from build123d import *

# Parameters (mm, degrees)
EXTRUDE_1_DEPTH     = 20
SKETCH_3_R          = 14
CUT_EXTRUDE_1_DEPTH = 20
SKETCH_4_R          = 3
CUT_EXTRUDE_2_DEPTH = 22.516585743
EXTRUDE_2_DEPTH     = 20
SKETCH_7_R          = 13.5
CUT_EXTRUDE_3_DEPTH = 28
SKETCH_8_R          = 3
CUT_EXTRUDE_4_DEPTH = 20
SKETCH_9_R          = 7.5
SKETCH_9_R_2        = 3
CUT_EXTRUDE_5_DEPTH = 20


# Read off the part's stored shape, not the designer's step: 填料-伸長1
with BuildPart() as part:
    # 填料-伸長1 outline → 填料-伸長1 (new body)
    with BuildSketch(Plane(origin=(0, 0, 0), x_dir=(0, 0, -1), z_dir=(1, 0, 0))):
        Polygon((-4019.675958787, 200.25160655), (-4018.512862627, 177.765080788), (-3958.59296353, 180.864385914), (-3959.75605969, 203.350911676), align=None)
    extrude(amount=EXTRUDE_1_DEPTH)

    # 草圖3 → 除料-伸長1 (cut)
    with BuildSketch(Plane.ZY):
        with Locations((3988.552913079, 179.314733351)):
            Circle(SKETCH_3_R)
    extrude(amount=-CUT_EXTRUDE_1_DEPTH, mode=Mode.SUBTRACT)

    # 草圖4 → 除料-伸長2 (cut)
    with BuildSketch(Plane(origin=(0, 407.076792548, 21.055696166), x_dir=(1, 0, 0), z_dir=(0, 0.9986649849421085, 0.051655085428040495))):
        with Locations(Location((10, -3950.965617011, 0), (0, 0, 270))):
            Circle(SKETCH_4_R)
    cut_extrude_2 = extrude(amount=-CUT_EXTRUDE_2_DEPTH, mode=Mode.SUBTRACT)

    # 鏡射1: 除料-伸長2 across plane
    add(cut_extrude_2.mirror(Plane(origin=(0, -205.275533435, 3968.660313072), x_dir=(1, 0, 0), z_dir=(0, 0.05165508542804326, -0.9986649849421085))), mode=Mode.SUBTRACT)


with BuildPart() as body_2:
    # 草圖6 → 填料-伸長2 (new body)
    with BuildSketch(Plane(origin=(0, 0, 0), x_dir=(0, 0, -1), z_dir=(1, 0, 0))):
        with BuildLine():
            Line((-4017.894989071, 165.819525376), (-4018.512862627, 177.765080788))
            Line((-4018.512862627, 177.765080788), (-3958.59296353, 180.864385914))
            Line((-3958.59296353, 180.864385914), (-3957.975089975, 168.918830502))
            ThreePointArc((-3957.975089975, 168.918830502), (-3987.51981137, 159.341433652), (-4017.894989071, 165.819525376))
        make_face()
    extrude(amount=EXTRUDE_2_DEPTH)

    # 草圖7 → 除料-伸長3 (cut)
    with BuildSketch(Plane.ZY):
        with Locations((3988.552913079, 179.314733351)):
            Circle(SKETCH_7_R)
    extrude(amount=-CUT_EXTRUDE_3_DEPTH, mode=Mode.SUBTRACT)

    # 草圖8 → 除料-伸長4 (cut)
    with BuildSketch(Plane(origin=(0, 384.590266786, 19.892600006), x_dir=(1, 0, 0), z_dir=(0, 0.9986649849421085, 0.05165508542804074))):
        with Locations(Location((10, -3996.965617011, 0), (0, 0, 270))):
            Circle(SKETCH_8_R)
    cut_extrude_4 = extrude(amount=-CUT_EXTRUDE_4_DEPTH, mode=Mode.SUBTRACT)

    # 草圖9 → 除料-伸長5 (cut)
    with BuildSketch(Plane(origin=(0, 372.644711374, 19.27472645), x_dir=(1, 0, 0), z_dir=(0, 0.9986649849421085, 0.05165508542804074))):
        with Locations((10, -3996.965617011)):
            Circle(SKETCH_9_R)
        with Locations(Location((10, -3996.965617011, 0), (0, 0, 270))):
            Circle(SKETCH_9_R_2, mode=Mode.SUBTRACT)
    cut_extrude_5 = extrude(amount=-CUT_EXTRUDE_5_DEPTH, mode=Mode.SUBTRACT)

    # 鏡射4: 除料-伸長4, 除料-伸長5 across plane
    add(cut_extrude_4.mirror(Plane(origin=(0, -205.275533435, 3968.660313072), x_dir=(1, 0, 0), z_dir=(0, 0.05165508542804326, -0.9986649849421085))), mode=Mode.SUBTRACT)
    add(cut_extrude_5.mirror(Plane(origin=(0, -205.275533435, 3968.660313072), x_dir=(1, 0, 0), z_dir=(0, 0.05165508542804326, -0.9986649849421085))), mode=Mode.SUBTRACT)


solid = body_2.part
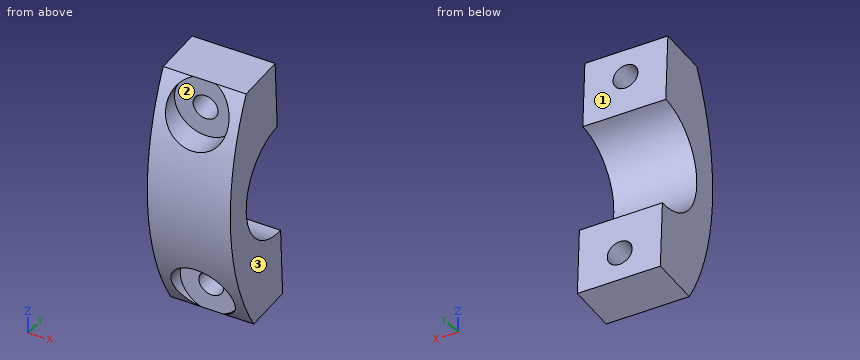
Could you check a few things on this model? Use its own coordinates, in mm. Face numbers are marked on the shaded views. Give positions to 0.01 mm unless a question says otherwise; leave off trailing zeros. Order: outer loops, then holes, each group sorted by start corner. A loop starts at its lowest first (then second) coordinate and runs counter-clockwise, first axis right, second up. Notation, with made-up numbers: (22.5, -2.5) -> (38.5, -2.5) arc R14 cw to (38.5, 18.5) -> close; hole circle Ø2 at (57.25, 5). An arc over 180 degrees is marked (long way). Answer in a Markdown table with one row per item. Add a question column.
Item 1: I'm going to push flat-ended pins straight in: P1, Ø10, axis at x = 8, z = 3983, coming from the -Y side; P2, Ø6, axis at x = 5.5, z = 3988, coming from the +Y side; P3, Ø1.5, axis at x = 11.5, y = 176, coming from the +Z side. Where does each tip first touch, or does it pass through?
Item 2: Imagine slicing it at C-C (z = 3980.5). List the corners of the cut face in (x, y) for me, and give its area (3 significant figures).
Item 3: Imagine slicing it at A-A (y = 173.5). Count the separate pieces of the cut face and the enclosed holes in it, and give its area (3 significant figures).
Item 4: Please list where these lines run through material, in increasing order: probe 1 along Z at (x, y) = (12.75, 175.5); probe 2 along Z at (x, y) = (12.75, 169); probe 3 along Z at (x, y) = (18.75, 175.75).
Item 5: We'd pull the mould along X, two halves only. Please class the marked faces 1, 2 and 3: pulls with the +X half, pulls with the -X half, needs draft (parallel to the pull), parting line crosses it, or undercut.
Result:
| question | item | result |
|---|---|---|
| 1 | P1 | y = 159.32 |
| 1 | P2 | y = 166.29 |
| 1 | P3 | z = 4018.46 |
| 2 | outline | (0, 160.12) -> (20, 160.12) -> (20, 168.48) -> (0, 168.48) -> close |
| 2 | area | 167 mm2 |
| 3 | separate pieces | 2 |
| 3 | enclosed holes | 2 |
| 3 | area | 658 mm2 |
| 4 | probe 1 | 3958.32 to 3964.12, 3966.53 to 3975.6, 4001.5 to 4010.19, 4012.59 to 4018.4 |
| 4 | probe 2 | 3957.98 to 3963.79, 3966.19 to 3979.84, 3997.26 to 4009.85, 4012.25 to 4018.06 |
| 4 | probe 3 | 3958.33 to 3975.53, 4001.57 to 4018.41 |
| 5 | face 1 | needs draft |
| 5 | face 2 | undercut |
| 5 | face 3 | pulls with the +X half |
